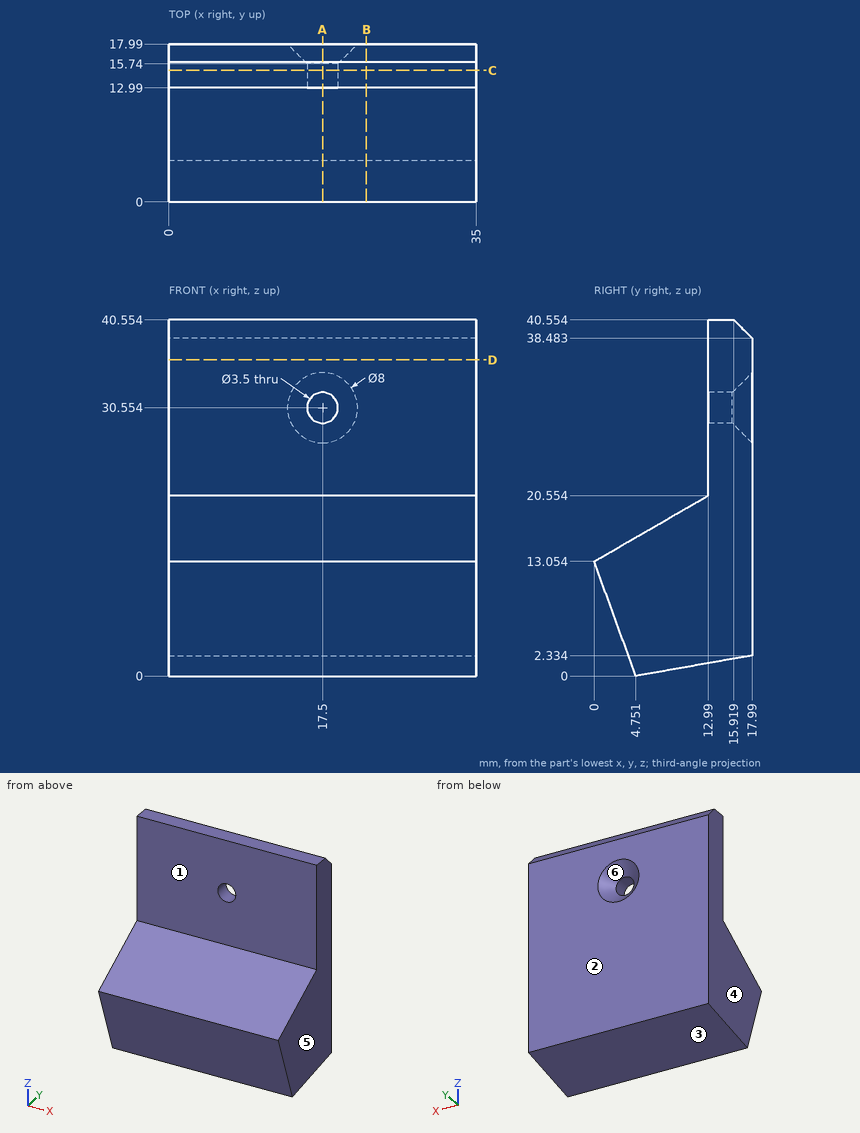
Check sheet for the drawn part. Datum: minimum x, y, z corner. Units: mm. A direction names the side the tool comes from. Round coordinates to 2 decimals unless told otherwise and drop trailing zeros. Loops run counter-clockwise (first coordinate to the right, second up) from the corner with the lowest first, then second, coordinate; pieces in that order, holes last. Notation, with made-up numbers: (-35, 43) -> (20, 43) arc R31 ccw to (20, 75) -> close; hole circle Ø4 at (51, 63.5). An arc over 180 degrees is marked (long way). Put each result on its own line as item: value. Start each with the question number.
1. Scan lines: probe 1 along Y at (x, z) = (12.5, 28); probe 2 along Z at (x, y) = (17.5, 14.35) (1 decimal); probe 3 along Z at (x, y) = (17.5, 14.95) (1 decimal). Record each from-to range of solid material in increasing order.
2. Section check C-C (y = 15). Enter the section's corners in (x, z).
3. Access from +Z, -Z, +X, -X, +Y, -Y to the whole of each face (thin tool, end or side, straight path). Record for the marked faces 1 and 2.
4. Gauge pin test, flat ends, axial feed: pin 1 (4 mm diameter, centred on x = 17, y = 14, fed in from -Z); pin 2 (1.5 mm diameter, centred on x = 23.5, z = 7.5, fed in from -Y); pin 3 (10 mm diameter, centred on x = 12.5, z = 33.5, fed in from -Y). Record the tip position at first contact, or that the pin passes through.
5. Draft check along X on the marked faces 3, 4, 5 and 6. Enter one of: +X half, -X half, draft (parallel to the pull), parting line (faces both ways), or undercut.
6. Section check A-A (x = 17.5). Enter the section's corners in (y, z) (1 decimal), plus the area to 3 significant figures.
7. Section check B-B (x = 22.5). Enter the section's corners in (y, z) (1 decimal).
8. Section check D-D (z = 36). Enter the section's corners in (x, y).
Findings:
1. probe 1: y = 12.99 to 17.99
1. probe 2: z = 1.7 to 28.8, 32.3 to 40.6
1. probe 3: z = 1.8 to 28.8, 32.3 to 40.6
2. outline: (0, 1.81) -> (35, 1.81) -> (35, 40.55) -> (0, 40.55) -> close; hole circle Ø3.5 at (17.5, 30.55)
3. face 1: +Z, +X, -X, -Y
3. face 2: +Z, -Z, +X, -X, +Y
4. pin 1: stops at z = 1.28
4. pin 2: stops at y = 1.75
4. pin 3: stops at y = 12.99
5. face 3: draft
5. face 4: -X half
5. face 5: +X half
5. face 6: undercut
6. outline: (0, 13.1) -> (4.8, 0) -> (18, 2.3) -> (18, 26.6) -> (15.7, 28.8) -> (13, 28.8) -> (13, 20.6) -> close; (13, 32.3) -> (15.7, 32.3) -> (18, 34.6) -> (18, 38.5) -> (15.9, 40.6) -> (13, 40.6) -> close
6. area: 350 mm^2
7. outline: (0, 13.1) -> (4.8, 0) -> (18, 2.3) -> (18, 38.5) -> (15.9, 40.6) -> (13, 40.6) -> (13, 20.6) -> close
8. outline: (0, 12.99) -> (35, 12.99) -> (35, 17.99) -> (0, 17.99) -> close
